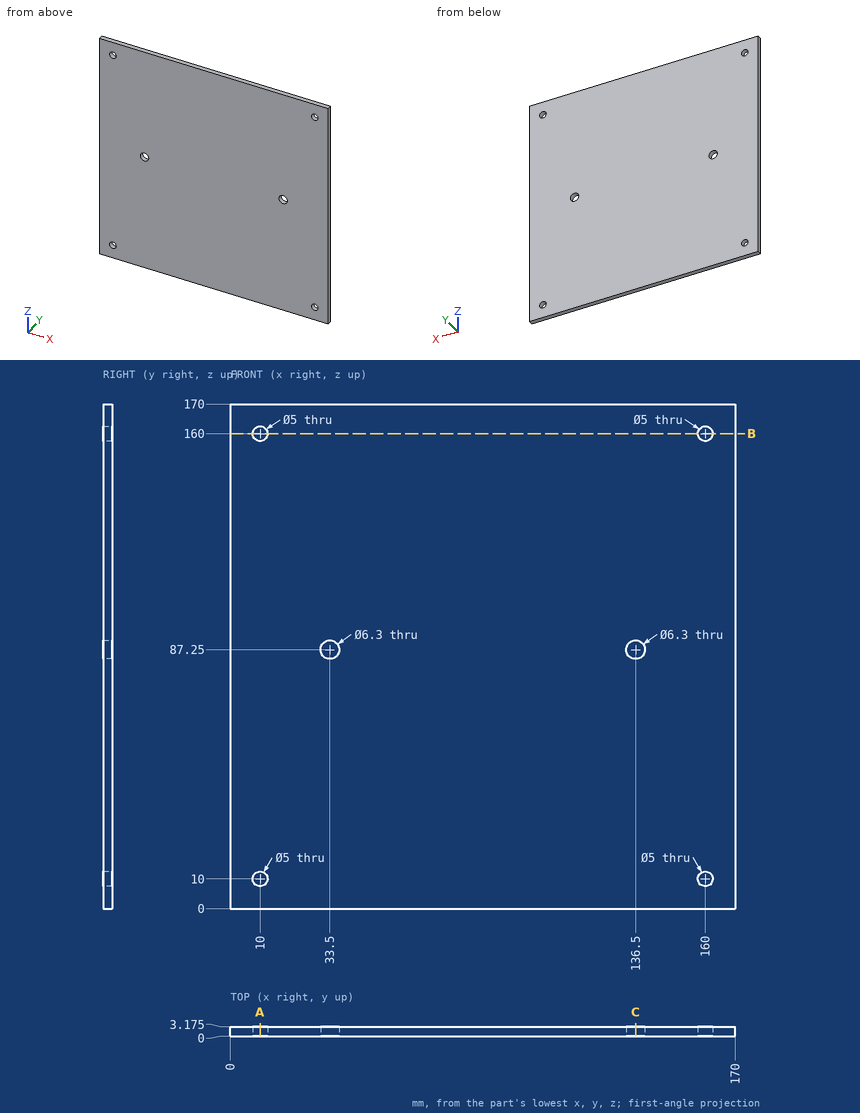
Could you check a few things on this drawing? It's one solid part, dimensions in mm from its lowest x, y, z. Round coordinates to 2 decimals unless told otherwise and drop trailing zeros. Loops run counter-clockwise (first coordinate to the right, second up) from the corner with the lowest first, then second, coordinate; pieces in that order, holes last.
Q1. I want a section at C-C (x = 136.5). Write out the boundary of the cut face in (y, z) (3 decimals).
Q2. I want a section at A-A (x = 10). Write out the boundary of the cut face in (y, z) (3 decimals).
Q3. Please list where these lines run through material, in increasing order: L1, parallel to X at y = 1.95, z = 87.25; L2, parallel to X at y = 2.25, z = 160.
Q4. I want a section at B-B (z = 160). Write out the boundary of the cut face in (x, y) (3 decimals).
Answer below:
1. outline: (0, 0) - (3.175, 0) - (3.175, 84.1) - (0, 84.1) - close; (0, 90.4) - (3.175, 90.4) - (3.175, 170) - (0, 170) - close
2. outline: (0, 0) - (3.175, 0) - (3.175, 7.5) - (0, 7.5) - close; (0, 12.5) - (3.175, 12.5) - (3.175, 157.5) - (0, 157.5) - close; (0, 162.5) - (3.175, 162.5) - (3.175, 170) - (0, 170) - close
3. L1: x = 0 to 30.35, 36.65 to 133.35, 139.65 to 170
3. L2: x = 0 to 7.5, 12.5 to 157.5, 162.5 to 170
4. outline: (0, 0) - (7.5, 0) - (7.5, 3.175) - (0, 3.175) - close; (12.5, 0) - (157.5, 0) - (157.5, 3.175) - (12.5, 3.175) - close; (162.5, 0) - (170, 0) - (170, 3.175) - (162.5, 3.175) - close
